Could you check a few things on this model? Use its own coordinates, in mm. Face numbers are marked on the shaded views. A direction names the side the tool comes from. Round coordinates to 2 decimals unless told otherwise and drop trailing zeros. Write each loop counter-clockwise with the first axis right and the second up, starting at its lowest first coordinate (ties: lowest second). Pieces come first, ordered by that corner, then holes. Notation, with made-up numbers: M 75.5,-11 L 113.5,-11 A23 cw 113.5,17 Z; hole C 9,30.25 d4. An arc over 180 degrees is marked long. One line per question, with ' | ' between items. Start each with the question number.
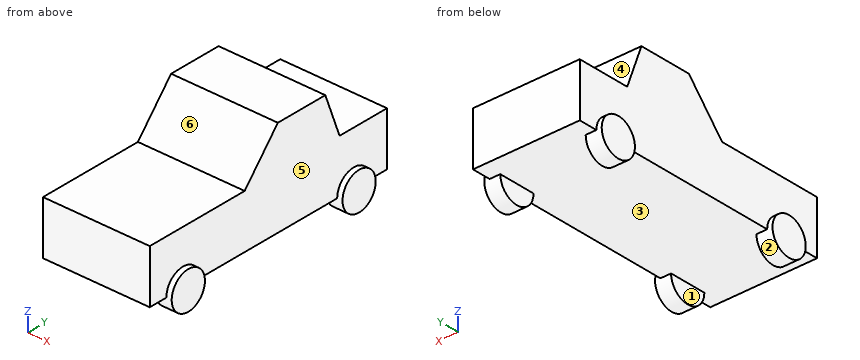
Autodesk Fusion 360 part; units mm, degrees
sketch "スケッチ1" plane through (0, 0, 0) normal (1, 0, 0) x (0, 1, 0)
  line L0 (0, 0) -> (0, 10)
  line L1 (0, 10) -> (20, 10)
  line L2 (20, 10) -> (20, 18)
  line L3 (20, 18) -> (40, 18)
  line L4 (40, 18) -> (40, 10)
  line L5 (40, 10) -> (50, 10)
  line L6 (50, 10) -> (50, 0)
  line L7 (50, 0) -> (0, 0)
  dimension "d1" = 10
  dimension "d2" = 10
  dimension "d3" = 20
  dimension "d4" = 8
  dimension "d5" = 10
  dimension "d6" = 20
extrude "押し出し1" add sketch "スケッチ1" along normal blind 20
sketch "スケッチ2" plane through (20, 0, 0) normal (1, 0, 0) x (0, 1, 0)
  line L0 (50, 0) -> (50, 10)
  line L1 (50, 10) -> (40, 10)
  line L2 (40, 10) -> (40, 18)
  line L3 (40, 18) -> (20, 18)
  line L4 (20, 18) -> (20, 10)
  line L5 (20, 10) -> (0, 10)
  line L6 (0, 10) -> (0, 0)
  line L7 (0, 0) -> (50, 0)
  circle A0 centre (7, 0) radius 3.5
  circle A1 centre (43, 0) radius 3.5
  dimension "d9" = 7
  dimension "d10" = 7
  dimension "d11" = 7
  dimension "d12" = 7
extrude "押し出し2" add sketch "スケッチ2" along normal blind 1 and the other way blind 2 contours L7 A1 | L7 A1 | L7 A0 | L7 A0
ref_plane "作業平面1" through (10, 25, 9) normal (1, 0, 0) x (0, 0, -1)
mirror "ミラー1" about plane through (10, 25, 9) normal (1, 0, 0) of "押し出し2"
sketch "スケッチ3" plane through (20, 0, 0) normal (1, 0, 0) x (0, 1, 0)
  arc A0 (46.5, 0) -> (39.5, 0) centre (43, 0) ccw
  line L0 (46.5, 0) -> (50, 0)
  line L1 (50, 0) -> (50, 10)
  line L2 (50, 10) -> (40, 10)
  line L3 (40, 10) -> (40, 18)
  line L4 (40, 18) -> (20, 18)
  line L5 (20, 18) -> (20, 10)
  line L6 (20, 10) -> (0, 10)
  line L7 (0, 10) -> (0, 0)
  line L8 (0, 0) -> (3.5, 0)
  arc A1 (10.5, 0) -> (3.5, 0) centre (7, 0) ccw
  line L9 (10.5, 0) -> (39.5, 0)
  line L10 (20, 10) -> (27, 18)
  line L11 (40, 10) -> (37, 18)
  dimension "d19" = 7
  dimension "d20" = 3
extrude "押し出し3" cut sketch "スケッチ3" against normal blind 20 contours L3 L4 L11 | L4 L5 L10
1. Which directions (+Z, -Z, +X, -X, +Y, -Y) give clear straight access to the entire face, cutting with the end or side of a thin tool? Please do the marked faces 1, 2 and 3.
2. Suppose I cut it at A-A (x = 10.25). Write out the boundary of the cut face in (y, z).
3. I need wall thicknesses on line 1 along Y through (x, z) = (1, -0.25); line 2 along Z through (x, y) = (15, 31); line 3 along Z through (x, y) = (5, 44.5). Which ranges of each line are inside material? Lowest first, please. Write a range as from..to.
4. Suppose I cut it at C-C (z = 4.5). Write out the boundary of the cut face in (x, y), and give its area (3 significant figures).
5. Suppose I cut it at D-D (y = 30). Write out the boundary of the cut face in (x, z).
6. I'm going to push flat-ended pins straight in: P1, Ø12, axis at y = 19.5, z = 6, coming from the -X side; P2, Ø2, axis at y = 37.5, z = 14, coming from the +X side; P3, Ø5, axis at x = 16, z = 14.5, coming from the -Y side. Where does each tip first touch, or does it pass through?
7. Suppose I cut it at B-B (y = 7). Write out the boundary of the cut face in (x, z), and give its area (3 significant figures).
8. If we mould it in two halves opening along Y, with no side actions, what happens to the marked faces 4, 5 and 6? For each: released by +Y, released by -Y, zero draft, split by the parting line, or undercut.
Computed:
1) face 1: -Z, +Y, -Y | face 2: -X | face 3: -Z
2) outline: M 0,0 L 50,0 L 50,10 L 40,10 L 37,18 L 27,18 L 20,10 L 0,10 Z
3) line 1: y = 3.51..10.49, 39.51..46.49 | line 2: z = 0..18 | line 3: z = 0..10
4) outline: M 0,0 L 20,0 L 20,50 L 0,50 Z | area: 1,000 mm²
5) outline: M 0,0 L 20,0 L 20,18 L 0,18 Z
6) P1: stops at x = 0 | P2: stops at x = 20 | P3: stops at y = 21.75
7) outline: M -1,-3.5 L 2,-3.5 L 2,0 L 18,0 L 18,-3.5 L 21,-3.5 L 21,3.5 L 20,3.5 L 20,10 L 0,10 L 0,3.5 L -1,3.5 Z | area: 228 mm²
8) face 4: released by +Y | face 5: undercut | face 6: released by -Y
